Verification items for the finished model (mm, model axes). A direction names the side the tool comes from. Give positions to 0.01 mm unless a question says otherwise; leave off trailing zeros. Write each loop counter-clockwise with the first axis right and the second up, starting at its lowest first coordinate (ties: lowest second). Pieces come first, ordered by that corner, then holes. Notation, with made-up numbers: M -7.75,8.5 L 2.25,8.5 A30 cw 2.25,43.5 Z; hole C 28,72.5 d1. An arc over 180 degrees is marked long. Answer as a JSON object with one key per item and string values.
```python
from build123d import *

# Parameters (mm, degrees)
SKETCH1_W                  = 109.5
SKETCH1_H                  = 83
BOSS_EXTRUDE1_DEPTH        = 2
F_3_2_3_2_DIAMETER_HOLE1_D = 3.2
F_2_2_2_2_DIAMETER_HOLE1_D = 2.2
SKETCH12_R                 = 3
CUT_EXTRUDE1_DEPTH         = 1
FILLET1_R                  = 3
FILLET2_R                  = 1


with BuildPart() as part:
    # Sketch1 → Boss-Extrude1 (new body)
    with BuildSketch(Plane.XY.offset(7.43465612)):
        with Locations((-0.743641502, 44.95185693)):
            Rectangle(SKETCH1_W, SKETCH1_H)
        with BuildLine():
            Line((-42.493641502, 80.45185693), (41.006358498, 80.45185693))
            ThreePointArc((41.006358498, 80.45185693), (43.127678842, 79.573177274), (44.006358498, 77.45185693))
            Line((44.006358498, 77.45185693), (44.006358498, 54.95185693))
            Line((44.006358498, 54.95185693), (48.006358498, 54.95185693))
            Line((48.006358498, 54.95185693), (48.006358498, 44.95185693))
            Line((48.006358498, 44.95185693), (48.006358498, 34.95185693))
            Line((48.006358498, 34.95185693), (44.006358498, 34.95185693))
            Line((44.006358498, 34.95185693), (44.006358498, 12.45185693))
            ThreePointArc((44.006358498, 12.45185693), (43.127678842, 10.330536587), (41.006358498, 9.45185693))
            Line((41.006358498, 9.45185693), (-42.493641502, 9.45185693))
            ThreePointArc((-42.493641502, 9.45185693), (-44.614961845, 10.330536587), (-45.493641502, 12.45185693))
            Line((-45.493641502, 12.45185693), (-45.493641502, 34.95185693))
            Line((-45.493641502, 34.95185693), (-49.493641502, 34.95185693))
            Line((-49.493641502, 34.95185693), (-49.493641502, 54.95185693))
            Line((-49.493641502, 54.95185693), (-45.493641502, 54.95185693))
            Line((-45.493641502, 54.95185693), (-45.493641502, 77.45185693))
            ThreePointArc((-45.493641502, 77.45185693), (-44.614961845, 79.573177274), (-42.493641502, 80.45185693))
        make_face(mode=Mode.SUBTRACT)
    extrude(amount=BOSS_EXTRUDE1_DEPTH)

    # Ø3.2 (3.2) Diameter Hole1 (through all)
    with Locations(Plane.XY.offset(9.43465612)):
        with Locations((-48.993641502, 6.95185693), (-48.993641502, 82.95185693), (47.506358498, 82.95185693), (47.506358498, 6.95185693)):
            Hole(F_3_2_3_2_DIAMETER_HOLE1_D / 2)

    # Ø2.2 (2.2) Diameter Hole1 (through all)
    with Locations(Plane(origin=(-25.493641502, 83.45185693, 9.43465612), x_dir=(1, 0, 0), z_dir=(0, 0, 1))):
        with Locations((0, 0), (49.5, 0), (49.5, -77), (0, -77)):
            Hole(F_2_2_2_2_DIAMETER_HOLE1_D / 2)

    # Sketch12 → Cut-Extrude1 (cut)
    with BuildSketch(Plane.XY.offset(9.43465612)):
        with Locations((-48.993641502, 82.95185693)):
            Circle(SKETCH12_R)
        with Locations((47.506358498, 82.95185693)):
            Circle(SKETCH12_R)
        with Locations((47.506358498, 6.95185693)):
            Circle(SKETCH12_R)
        with Locations((-48.993641502, 6.95185693)):
            Circle(SKETCH12_R)
    extrude(amount=-CUT_EXTRUDE1_DEPTH, mode=Mode.SUBTRACT)

    # Fillet1
    fillet1_edges = [part.edges().sort_by_distance(p)[0] for p in [
        (48.006358498, 34.95185693, 8.43465612),
        (48.006358498, 54.95185693, 8.43465612),
        (-49.493641502, 54.95185693, 8.43465612),
        (-49.493641502, 34.95185693, 8.43465612),
    ]]
    fillet(fillet1_edges, radius=FILLET1_R)

    # Fillet2
    fillet2_edges = [part.edges().sort_by_distance(p)[0] for p in [
        (44.006358498, 34.95185693, 8.43465612),
        (44.006358498, 54.95185693, 8.43465612),
        (-45.493641502, 34.95185693, 8.43465612),
        (-45.493641502, 54.95185693, 8.43465612),
    ]]
    fillet(fillet2_edges, radius=FILLET2_R - 0.0001)  # a hair under: the kernel refuses the full size


solid = part.part
```
1) Section check B-B on x = -8. Record the boundary of the cut face in (y, z), and give its area (3 significant figures).
Completed:
{"outline": "M 3.45,7.43 L 9.45,7.43 L 9.45,9.43 L 3.45,9.43 Z; M 80.45,7.43 L 86.45,7.43 L 86.45,9.43 L 80.45,9.43 Z", "area": "24.0 mm2"}
2) Go/stop test with a flat-tipped pin: pin 1 (5.5 mm diameter, centred on x = -48.99, y = 6.95, fed in from +Z). Record where the tip stops, or that it passes through.
Completed:
{"pin 1": "stops at z = 8.43"}
3) Access from +Z, -Z, +X, -X, +Y, -Y to the whole of each face (thin tool, end or side, straight path). Record for faces 1 (the face through (-5, 8, 7.435)), 2 (the face through (44.51, 7.08, 8.94)), 3 (the face through (-48.638, 35.854, 8.449)).
Completed:
{"face 1": "-Z, +X, -X, +Y, -Y", "face 2": "+Z", "face 3": "+Z, -Z"}
4) Thickness scan on L1, parallel to X at y = 43, z = 9.2; L2, parallel to X at y = 74.5, z = 8.55; L3, parallel to Y at x = -40, z = 9.15. Record the ranges inside material, lowest first.
Completed:
{"L1": "x = -55.49 to -49.49, 48.01 to 54.01", "L2": "x = -55.49 to -45.49, 44.01 to 54.01", "L3": "y = 3.45 to 9.45, 80.45 to 86.45"}
5) Section check A-A on y = 60.5. Record the boundary of the cut face in (x, z).
Completed:
{"outline": "M -55.49,7.43 L -45.49,7.43 L -45.49,9.43 L -55.49,9.43 Z; M 44.01,7.43 L 54.01,7.43 L 54.01,9.43 L 44.01,9.43 Z"}
6) Section check C-C on z = 9. Count the separate pieces of the cut face and the enclosed holes in it, and give its area (3 significant figures).
Completed:
{"separate pieces": "1", "enclosed holes": "9", "area": "2,460 mm2"}
7) Release check for a two-part mould opening along X. For faces 4 (the face through (-51.205, 84.979, 8.942)), 5 (the face through (-5, 8, 9.435)) record: pulls with the +X half, pulls with the -X half, needs draft (parallel to the pull), parting line crosses it, or undercut.
Completed:
{"face 4": "undercut", "face 5": "needs draft"}
